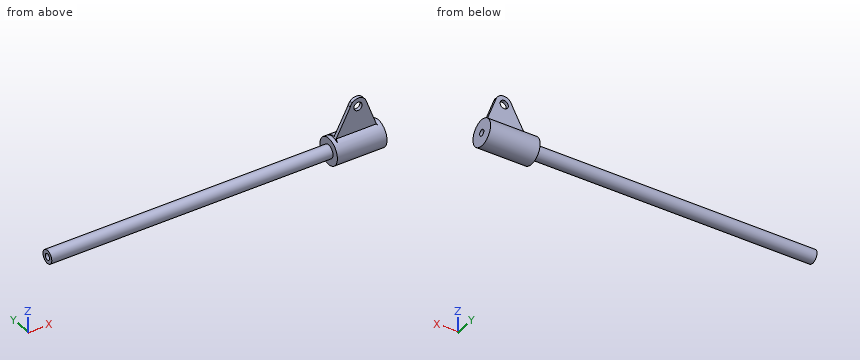
from build123d import *

# Parameters (mm, degrees)
SKETCH8_W               = 245.440082446
SKETCH8_H               = 20
BOSS_EXTRUDE1_DEPTH     = 400
CUT_EXTRUDE8_DEPTH      = 1704.211489704
CUT_EXTRUDE8_DEPTH_BACK = 1704.211489704
SKETCH9_R               = 25
CUT_EXTRUDE9_DEPTH      = 1679.423730942
CUT_EXTRUDE9_DEPTH_BACK = 1679.423730942
SKETCH10_R              = 19.05


with BuildPart() as part:
    # Sketch2 → Revolve1 (revolve)
    with BuildSketch(Plane.XY, mode=Mode.PRIVATE) as revolve1_sk:
        Polygon((1650, -24.245152355), (1350, -24.245152355), (1350, 15.754847645), (-350, 15.754847645), (-350, 55.754847645), (1650, 55.754847645), align=None)
    revolve(revolve1_sk.sketch.rotate(Axis((1650, 55.754847645, 0), (-1, 0, 0)), 180), axis=Axis((1650, 55.754847645, 0), (-1, 0, 0)))

    # Sketch8 → Boss-Extrude1 (add)
    with BuildSketch(Plane.XY):
        with Locations((1502.581339025, 43.148524262)):
            Rectangle(SKETCH8_W, SKETCH8_H)
    extrude(amount=BOSS_EXTRUDE1_DEPTH)

    # Sketch9 → Cut-Extrude8 (cut, two sides: drawn at the far end of the back side and taken through both)
    with BuildSketch(Plane(origin=(0, 0, 0), x_dir=(1, 0, 0), z_dir=(0, 1, 0)).offset(-CUT_EXTRUDE8_DEPTH_BACK)):
        with BuildLine():
            ThreePointArc((1561.210933041, -243.569878217), (1523.352220911, -275.193400776), (1476.779097647, -258.936911225))
            ThreePointArc((1476.779097647, -258.936911225), (1470.218517898, -249.41265784), (1466.021642395, -238.635884427))
            Line((1466.021642395, -238.635884427), (1374.277655751, -65.500408808))
            Line((1374.277655751, -65.500408808), (1374.277655751, -447.060346657))
            Line((1374.277655751, -447.060346657), (1625.633642708, -447.060346657))
            Line((1625.633642708, -447.060346657), (1625.633642708, -71.911854778))
            Line((1625.633642708, -71.911854778), (1561.210933041, -243.569878217))
        make_face()
        with Locations(Location((1512.641248766, -225.471244951, 0), (0, 0, 270))):
            Circle(SKETCH9_R)
    extrude(amount=CUT_EXTRUDE8_DEPTH + CUT_EXTRUDE8_DEPTH_BACK, mode=Mode.SUBTRACT)

    # Sketch10 → Cut-Extrude9 (cut, two sides: drawn at the far end of the back side and taken through both)
    with BuildSketch(Plane(origin=(0, 0, 0), x_dir=(0, 0, -1), z_dir=(1, 0, 0)).offset(-CUT_EXTRUDE9_DEPTH_BACK)):
        with Locations((0, 55.754847645)):
            Circle(SKETCH10_R)
    extrude(amount=CUT_EXTRUDE9_DEPTH + CUT_EXTRUDE9_DEPTH_BACK, mode=Mode.SUBTRACT)


solid = part.part
Work out the finished part from the listing and answer in its coordinate system (mm). Round coordinates to 2 decimals unless told otherwise and drop trailing zeros. Write each loop counter-clockwise with the first axis right and the second up, starting at its lowest first coordinate (ties: lowest second). Pieces come first, ordered by that corner, then holes.
1) Straight lines are drawn through the part: line 1 (Z direction, x = 146.5, y = 59); line 2 (X direction, y = 55, z = 79); line 3 (Y direction, x = 522, z = -17). For each, find the intervals that lie inside material, in ascending order.
2) A cutting plane is placed at C-C (z = 152). Give the vertices of the cut face in (x, y).
3) Given pin 1 Ø3 at (x, z) = (1148.5, 29) entering from -Y; pin 2 Ø10 at (y, z) = (90.5, 78.5) entering from -X; pin 3 Ø2 at (y, z) = (36, 145.5) entering from -X; pin 4 Ø12 at (x, z) = (673.5, 7.5) entering from -Y, each flat-ended and moving along its own axis, determine where each tip first touches the part or whether it passes through.
4) A cutting plane is placed at B-B (x = 1213.5). Give the vertices of the cut face in (y, z).
5) A cutting plane is placed at A-A (z = 0). Give the vertices of the cut face in (x, y).
Completed:
1. line 1: z = -39.87 to -18.77, 18.77 to 39.87
1. line 2: x = 1350 to 1374.28, 1381.43 to 1622.97, 1625.63 to 1650
1. line 3: y = 19.55 to 47.16, 64.35 to 91.96
2. outline: (1420.11, 33.15) - (1595.58, 33.15) - (1595.58, 53.15) - (1420.11, 53.15) - close
3. pin 1: stops at y = 26.71
3. pin 2: passes through
3. pin 3: stops at x = 1416.14
3. pin 4: stops at y = 15.78
4. outline: circle Ø80 at (55.75, 0); hole circle Ø38.1 at (55.75, 0)
5. outline: (-350, 15.75) - (1350, 15.75) - (1350, -24.25) - (1650, -24.25) - (1650, 36.7) - (-350, 36.7) - close; (-350, 74.8) - (1650, 74.8) - (1650, 135.75) - (1350, 135.75) - (1350, 95.75) - (-350, 95.75) - close
